```python
from build123d import *

# Parameters (mm, degrees)
SKETCH1_R           = 3.75
BOSS_EXTRUDE1_DEPTH = 11.9
SKETCH2_R           = 3.75
SKETCH2_R_2         = 1.25
CUT_EXTRUDE1_DEPTH  = 10.2
FILLET1_R           = 0.6
CUT_EXTRUDE2_DEPTH  = 0.3


with BuildPart() as part:
    # Sketch1 → Boss-Extrude1 (new body)
    with BuildSketch(Plane.XY):
        Circle(SKETCH1_R)
    extrude(amount=BOSS_EXTRUDE1_DEPTH)

    # Sketch2 → Cut-Extrude1 (cut)
    with BuildSketch(Plane.XY.offset(11.9)):
        Circle(SKETCH2_R)
        Circle(SKETCH2_R_2, mode=Mode.SUBTRACT)
    extrude(amount=-CUT_EXTRUDE1_DEPTH, mode=Mode.SUBTRACT)

    # Fillet1
    fillet1_edges = [part.edges().sort_by_distance(p)[0] for p in [
        (-3.75, 0, 0),
    ]]
    fillet(fillet1_edges, radius=FILLET1_R)

    # Sketch3 → Cut-Extrude2 (cut)
    with BuildSketch(Plane.XY.offset(11.5)):
        with BuildLine():
            Line((0, 0.466411964), (-0.73212486, 1.013160002))
            ThreePointArc((-0.73212486, 1.013160002), (-1.25, 0), (-0.73212486, -1.013160002))
            Line((-0.73212486, -1.013160002), (0, -0.466411964))
            Line((0, -0.466411964), (0, 0.466411964))
        make_face()
    extrude(amount=-CUT_EXTRUDE2_DEPTH, mode=Mode.SUBTRACT)


solid = part.part
```
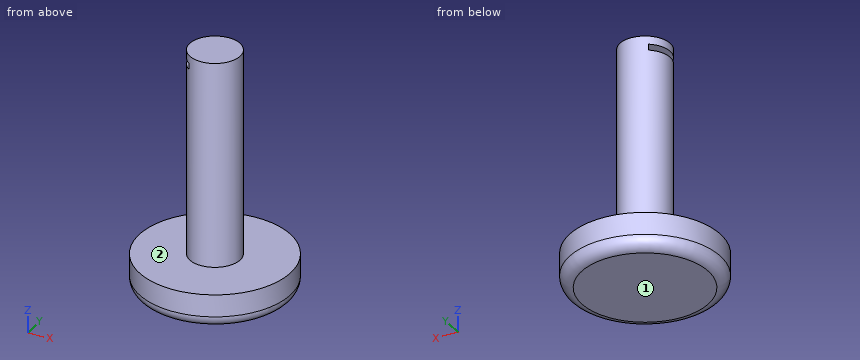
Could you check a few things on this model? Use its own coordinates, in mm. Face numbers are marked on the shaded views. A direction names the side the tool comes from. Round coordinates to 2 decimals unless told otherwise and drop trailing zeros. Write each loop counter-clockwise with the first axis right and the second up, starting at its lowest first coordinate (ties: lowest second). Pieces come first, ordered by that corner, then holes.
(1) For pin 1 (1 mm diameter, centred on x = -2.5, y = -1.5, fed in from +Z); pin 2 (1 mm diameter, centred on x = -0.5, y = -0.5, fed in from -Z); pin 3 (1 mm diameter, centred on x = 0, z = 5, fed in from -Y), each with a flat end and sliding along its axis, tell me the tip position at first contact or that it passes through.
Findings below:
pin 1: stops at z = 1.7
pin 2: stops at z = 0
pin 3: stops at y = -1.25
(2) Suppose I cut it at A-A on z = 2.5. Write out the boundary of the cut face in (x, y).
Findings below:
outline: circle Ø2.5 at (0, 0)
(3) Which directions (+Z, -Z, +X, -X, +Y, -Y) give clear straight access to the entire face, cutting with the end or side of a thin tool? Please do the marked faces 1 and 2.
Findings below:
face 1: -Z, +X, -X, +Y, -Y
face 2: +Z
(4) If I drill on probe 1 along Z at (x, y) = (-1.5, 0.75); probe 2 along X at (y, z) = (-0.5, 4.5); probe 3 along Y at (x, z) = (1, 2.25), over which ranges is the centre line in solid material (lowest first)?
Findings below:
probe 1: z = 0 to 1.7
probe 2: x = -1.15 to 1.15
probe 3: y = -0.75 to 0.75
